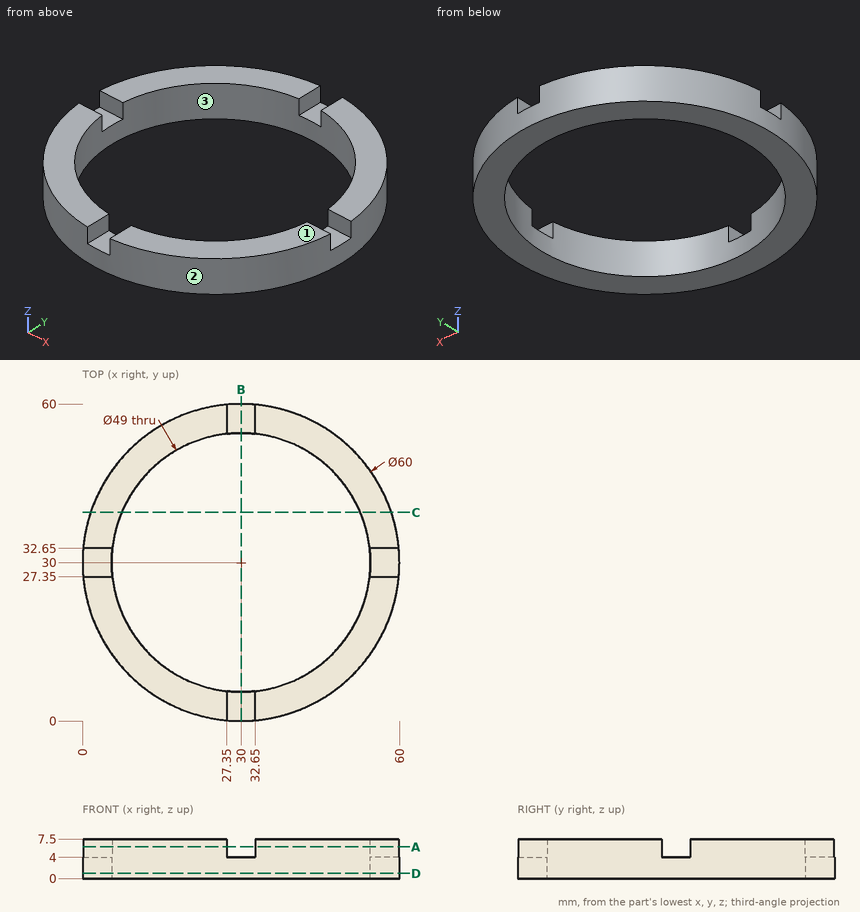
Part print with two shaded views. Sizes in mm from the minimum x, y, z corner. Give positions to 0.01 mm unless a question says otherwise; leave off trailing zeros. Order: outer loops, then holes, each group sorted by start corner. A loop starts at its lowest first (then second) coordinate and runs counter-clockwise, first axis right, second up.
1) Mould opens along X. For the marked faces 1, 2 and 3 say: +X half, -X half, draft (parallel to the pull), parting line (faces both ways), or undercut.
2) Saw through at B-B, the plane x = 30. Write the cut outline in (y, z), then the cut area to 3 significant figures.
3) Saw through at C-C, the plane y = 39.5. Write the cut outline in (x, z).
4) Wall check: probe 1 along Y at (x, z) = (30, 3.5); probe 2 along Y at (x, z) = (34, 5). Give the ranges that are in metal, low to high.
5) Saw through at A-A, the plane z = 6. Write the cut outline in (x, y).
6) Saw through at D-D, the plane z = 1. Write the cut outline in (x, y), then the cut area to 3 significant figures.
7) Pin check, flat tips, straight feed: pin 1 (1.8 mm diameter, centred on x = 58, z = 6, fed in from -Y); pin 2 (4 mm diameter, centred on x = 7, y = 26.5, fed in from +Z); pin 3 (4 mm diameter, centred on x = 2.5, z = 5.5, fed in from -Y); pin 4 (1.8 mm diameter, centred on x = 3, z = 5, fed in from +Y). Stop position of each tip, or through.
Computed:
1. face 1: draft
1. face 2: parting line
1. face 3: undercut
2. outline: (0, 0) - (5.5, 0) - (5.5, 4) - (0, 4) - close; (54.5, 0) - (60, 0) - (60, 4) - (54.5, 4) - close
2. area: 44.0 mm2
3. outline: (1.54, 0) - (7.42, 0) - (7.42, 7.5) - (1.54, 7.5) - close; (52.58, 0) - (58.46, 0) - (58.46, 7.5) - (52.58, 7.5) - close
4. probe 1: y = 0 to 5.5, 54.5 to 60
4. probe 2: y = 0.27 to 5.83, 54.17 to 59.73
5. outline: (0.12, 27.35) arc R30 ccw to (27.35, 0.12) - (27.35, 5.64) arc R24.5 cw to (5.64, 27.35) - close; (0.12, 32.65) - (5.64, 32.65) arc R24.5 cw to (27.35, 54.36) - (27.35, 59.88) arc R30 ccw to start; (32.65, 0.12) arc R30 ccw to (59.88, 27.35) - (54.36, 27.35) arc R24.5 cw to (32.65, 5.64) - close; (32.65, 54.36) arc R24.5 cw to (54.36, 32.65) - (59.88, 32.65) arc R30 ccw to (32.65, 59.88) - close
6. outline: circle Ø60 at (30, 30); hole circle Ø49 at (30, 30)
6. area: 942 mm2
7. pin 1: stops at y = 17.13
7. pin 2: stops at z = 7.5
7. pin 3: stops at y = 14.2
7. pin 4: stops at y = 44.79
